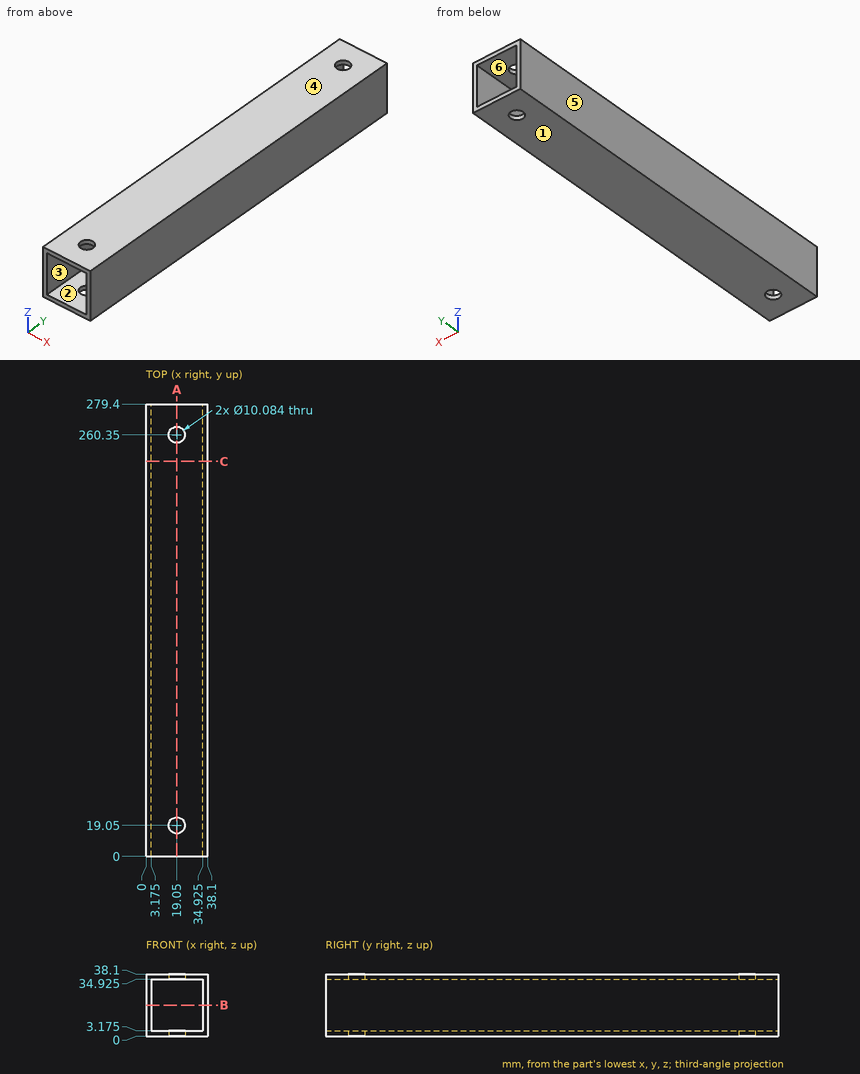
Part print with two shaded views. Sizes in mm from the minimum x, y, z corner. A direction names the side the tool comes from. Round coordinates to 2 decimals unless told otherwise and drop trailing zeros. Order: outer loops, then holes, each group sorted by start corner. A loop starts at its lowest first (then second) coordinate and runs counter-clockwise, first axis right, second up. Notation, with made-up numbers: (45, 14.25) -> (53, 14.25) arc R27 cw to (53, 33.25) -> close; hole circle Ø5 at (62.25, -39.5). An arc over 180 degrees is marked (long way). Write each question's results on one line, items separated by ' | '.
1. 3-axis set-ups, long thin cutter, end or side, ignore diameter. For the marked faces 1 and 2: which of +Z, -Z, +X, -X, +Y, -Y reach the whole face in a straight line?
Findings below:
face 1: -Z, +X, -X, +Y, -Y | face 2: +Y, -Y
2. Wall check: line 1 along Y through (x, z) = (19.05, 36.35); line 2 along X through (y, z) = (121.5, 21.5) (3 decimals). Give the ranges that are in metal, low to high. Write a range as [from, to].
Findings below:
line 1: y = [0, 14.01], [24.09, 255.31], [265.39, 279.4] | line 2: x = [0, 3.175], [34.925, 38.1]
3. Cut at C-C (y = 244). Give the cut face in (x, z) (3 decimals).
Findings below:
outline: (0, 0) -> (38.1, 0) -> (38.1, 38.1) -> (0, 38.1) -> close; hole (3.175, 3.175) -> (34.925, 3.175) -> (34.925, 34.925) -> (3.175, 34.925) -> close
4. Cut at B-B (z = 19). Give the cut face in (x, y) (3 decimals), plus the area to 3 significant figures.
Findings below:
outline: (0, 0) -> (3.175, 0) -> (3.175, 279.4) -> (0, 279.4) -> close; (34.925, 0) -> (38.1, 0) -> (38.1, 279.4) -> (34.925, 279.4) -> close | area: 1,770 mm²
5. Pull direction X, two halves, no side cores. Call the marked faces 3, 4, 5 and 6: pulls with the +X half, pulls with the -X half, needs draft (parallel to the pull), parting line crosses it, or undercut.
Findings below:
face 3: undercut | face 4: needs draft | face 5: pulls with the -X half | face 6: undercut
6. Cut at A-A (x = 19.05). Give the cut face in (y, z) (1 decimal).
Findings below:
outline: (0, 0) -> (14, 0) -> (14, 3.2) -> (0, 3.2) -> close; (0, 34.9) -> (14, 34.9) -> (14, 38.1) -> (0, 38.1) -> close; (24.1, 0) -> (255.3, 0) -> (255.3, 3.2) -> (24.1, 3.2) -> close; (24.1, 34.9) -> (255.3, 34.9) -> (255.3, 38.1) -> (24.1, 38.1) -> close; (265.4, 0) -> (279.4, 0) -> (279.4, 3.2) -> (265.4, 3.2) -> close; (265.4, 34.9) -> (279.4, 34.9) -> (279.4, 38.1) -> (265.4, 38.1) -> close
